from build123d import *

# Parameters (mm, degrees)
SKETCH_1_W          = 50
SKETCH_1_H          = 20
EXTRUDE_1_DEPTH     = 350
SKETCH_2_W          = 46
SKETCH_2_H          = 16
CUT_EXTRUDE_1_DEPTH = 352.034186369
SKETCH_3_R          = 4.5
CUT_EXTRUDE_3_DEPTH = 352.461235416


with BuildPart() as part:
    # Эскиз1 → Бобышка-Вытянуть1 (new body)
    with BuildSketch(Plane.XY):
        Rectangle(SKETCH_1_W, SKETCH_1_H)
    extrude(amount=EXTRUDE_1_DEPTH)

    # Эскиз2 → Вырез-Вытянуть1 (cut, through all)
    with BuildSketch(Plane.XY.offset(350)):
        Rectangle(SKETCH_2_W, SKETCH_2_H)
    extrude(amount=-CUT_EXTRUDE_1_DEPTH, mode=Mode.SUBTRACT)

    # Эскиз3 → Вырез-Вытянуть3 (cut, through all)
    with BuildSketch(Plane(origin=(0, 10, 0), x_dir=(-1, 0, 0), z_dir=(0, 1, 0))):
        with Locations(Location((-15, 325, 0), (0, 0, 90))):
            Circle(SKETCH_3_R)
        with Locations(Location((15, 325, 0), (0, 0, 90))):
            Circle(SKETCH_3_R)
        with Locations(Location((-15, 25, 0), (0, 0, 90))):
            Circle(SKETCH_3_R)
        with Locations(Location((15, 25, 0), (0, 0, 90))):
            Circle(SKETCH_3_R)
        with Locations(Location((-15, 160, 0), (0, 0, 90))):
            Circle(SKETCH_3_R)
        with Locations(Location((-15, 190, 0), (0, 0, 90))):
            Circle(SKETCH_3_R)
        with Locations(Location((15, 190, 0), (0, 0, 90))):
            Circle(SKETCH_3_R)
        with Locations(Location((15, 160, 0), (0, 0, 90))):
            Circle(SKETCH_3_R)
    extrude(amount=-CUT_EXTRUDE_3_DEPTH, mode=Mode.SUBTRACT)


solid = part.part
Verification items for the finished model (mm, model axes). A direction names the side the tool comes from. Round coordinates to 2 decimals unless told otherwise and drop trailing zeros. Loops run counter-clockwise (first coordinate to the right, second up) from the corner with the lowest first, then second, coordinate; pieces in that order, holes last. Notation, with made-up numbers: (55, 15) - (82, 15) arc R11 cw to (82, 25) - close; hole circle Ø8 at (36.25, 71). An arc over 180 degrees is marked (long way). Use one line per item in the form item = value.
1. Access from +Z, -Z, +X, -X, +Y, -Y to the whole of each face (thin tool, end or side, straight path). Record for faces 4 (the flat face through (0, -8, 177)), 5 (the cylindrical face through (16.352, 9.014, 329.292)).
A:
face_4 = +Z, -Z
face_5 = +Y, -Y
2. Section check C-C on x = 4.5. Record the cut outline in (y, z), and give its area (3 significant figures).
A:
outline = (-10, 0) - (-8, 0) - (-8, 350) - (-10, 350) - close; (8, 0) - (10, 0) - (10, 350) - (8, 350) - close
area = 1,400 mm²
3. Draft check along Y on faces 1 (the cylindrical face through (-13.648, 9.014, 329.292)), 2 (the flat face through (0, 10, 173)), 3 (the flat face through (0, 8, 177)). Enter one of: pulls with the +Y half, pulls with the -Y half, needs draft (parallel to the pull), parting line crosses it, or undercut.
A:
face_1 = needs draft
face_2 = pulls with the +Y half
face_3 = undercut
4. Gauge pin test, flat ends, axial feed: pin 1 Ø8 at (x, z) = (15, 25) entering from +Y (3 decimals); pin 2 Ø4 at (x, y) = (9.5, 6.5) entering from +Z. Record the tip position at first contact, or that the pin passes through.
A:
pin_1 = through
pin_2 = 350
5. Scan lines: probe 1 along X at (y, z) = (8.8, 325); probe 2 along X at (y, z) = (6.5, 133.5); probe 3 along Y at (x, z) = (-20.5, 203). Record each from-to range of solid material in increasing order.
A:
probe_1 = -25 to -19.5, -10.5 to 10.5, 19.5 to 25
probe_2 = -25 to -23, 23 to 25
probe_3 = -10 to -8, 8 to 10
6. Section check B-B on z = 325. Record the cut outline in (x, y), and give its area (3 significant figures).
A:
outline = (-25, -10) - (-19.5, -10) - (-19.5, -8) - (-23, -8) - (-23, 8) - (-19.5, 8) - (-19.5, 10) - (-25, 10) - close; (-10.5, -10) - (10.5, -10) - (10.5, -8) - (-10.5, -8) - close; (-10.5, 8) - (10.5, 8) - (10.5, 10) - (-10.5, 10) - close; (19.5, -10) - (25, -10) - (25, 10) - (19.5, 10) - (19.5, 8) - (23, 8) - (23, -8) - (19.5, -8) - close
area = 192 mm²
7. Section check A-A on y = 4.75. Record the cut outline in (x, z), and give its area (3 significant figures).
A:
outline = (-25, 0) - (-23, 0) - (-23, 350) - (-25, 350) - close; (23, 0) - (25, 0) - (25, 350) - (23, 350) - close
area = 1,400 mm²
